Part model, mm, in its own coordinate system. A direction names the side the tool comes from. Coordinates: 2 decimals unless noted, no trailing zeros. Loops run counter-clockwise (first coordinate to the right, second up) from the corner with the lowest first, then second, coordinate; pieces in that order, holes last. Notation, with made-up numbers: M 72,22.5 L 119,22.5 A29 cw 119,46.5 Z; hole C 20.5,55 d11. An arc over 180 degrees is marked long. Use a Markdown table: item, result. Add a question column.
1) Band-saw the part on B-B (z = 0). State how many separate pieces and enclosed holes the cut face has, plus the area to 3 significant figures.
2) Band-saw the part on C-C (x = 6). List the corners of the cut face in (y, z) (3 decimals).
3) Tool access for faces 5 (the flat face through (-6.2, 8.094, 1.2)), 6 (the flat face through (-10, -3, 2)), 7 (the flat face through (1.3, 16, 13)), 8 (the cylindrical face through (0.659, 13.143, -17.141)), 9 (the flat face through (0, 9, 0)): list every direction of +Z, -Z, +X, -X, +Y, -Y with a clear straight run to the whole face (end or side of a thin tool).
4) Band-saw the part on A-A (x = -5). List the corners of the cut face in (y, z) (3 decimals).
5) Wall check: probe 1 along Y at (x, z) = (-3, 0) (3 decimals); probe 2 along X at (y, z) = (6.9, 0); probe 3 along Y at (x, z) = (1.5, 0) (3 decimals). Give the ranges that are in metal, low to high. Write a range as from..to.
6) Pull direction Z, two halves, no side cores. Call faces 1 (the cylindrical face through (21.659, 13.143, -17.141)), 2 (the conical face through (23.146, 3.144, -0.698)), 3 (the flat face through (22.3, 16, 13)), 4 (the cylindrical face through (-4.55, 5.43, 1.43)): released by +Z, released by -Z, zero draft, split by the parting line, or undercut.
7) Pin check, flat tips, straight feed: pin 1 Ø3.5 at (x, z) = (-5, 0) entering from +Y; pin 2 Ø3 at (x, y) = (8, 10.5) entering from -Z; pin 3 Ø5 at (y, z) = (-15.5, -16) entering from -X; pin 4 Ø5 at (y, z) = (0, 0) entering from +X. Stop position of each tip, or through.
from build123d import *

# Parameters (mm, degrees)
FILLET3_R               = 8
FILLET4_R               = 8
SKETCH3_W               = 12
SKETCH3_H               = 3.642473792
CUT_EXTRUDE1_DEPTH      = 10
CUT_EXTRUDE2_REACH      = 46.992
CUT_EXTRUDE2_END_RADIUS = 3.075
SKETCH4_R               = 1.5
CHAMFER1_SIZE           = 3


with BuildPart() as part:
    # Sketch1 → Revolve1 (revolve)
    with BuildSketch(Plane.XY, mode=Mode.PRIVATE) as revolve1_sk:
        Polygon((0, 21.6), (1.3, 21.6), (1.3, 20.2), (3.7, 20.2), (3.7, 21.6), (5, 21.6), (5, 13.075), (21, 13.075), (21, 21.6), (22.3, 21.6), (22.3, 20.2), (24.7, 20.2), (24.7, 21.6), (26, 21.6), (26, 3.075), (-10, 3.075), (-10, 10.075), (0, 10.075), align=None)
    revolve(revolve1_sk.sketch.rotate(Axis((0, 0, 0), (1, 0, 0)), 90), axis=Axis((0, 0, 0), (1, 0, 0)))

    # Fillet3
    fillet3_edges = [part.edges().sort_by_distance(p)[0] for p in [
        (5, 0, -13.075),
    ]]
    fillet(fillet3_edges, radius=FILLET3_R)

    # Fillet4
    fillet4_edges = [part.edges().sort_by_distance(p)[0] for p in [
        (21, 0, -13.075),
    ]]
    fillet(fillet4_edges, radius=FILLET4_R - 0.0001)  # a hair under: the kernel refuses the full size

    # Sketch3 → Cut-Extrude1 (cut)
    with BuildSketch(Plane.ZY.offset(10)):
        with Locations((0, 9.91479143)):
            Rectangle(SKETCH3_W, SKETCH3_H)
    extrude(amount=-CUT_EXTRUDE1_DEPTH, mode=Mode.SUBTRACT)

    # Cut-Extrude2: up to this cylinder (the profile starts outside it)
    cut_extrude2_end = Plane(origin=(-5, 0, 0), z_dir=(-1, 0, 0)) * Cylinder(CUT_EXTRUDE2_END_RADIUS, 101.134, mode=Mode.PRIVATE)
    # Sketch4 → Cut-Extrude2 (cut, up to the surface)
    with BuildSketch(Plane(origin=(0, 8.093554534, 0), x_dir=(1, 0, 0), z_dir=(0, 1, 0)), mode=Mode.PRIVATE) as cut_extrude2_sk1:
        with Locations(Location((-5, 0, 0), (0, 0, 270))):
            Circle(SKETCH4_R)
    cut_extrude2_tool1 = extrude(cut_extrude2_sk1.sketch, amount=-CUT_EXTRUDE2_REACH, mode=Mode.PRIVATE) - cut_extrude2_end
    add(cut_extrude2_tool1.solids().sort_by_distance((-5, 8.093555, 0))[0], mode=Mode.SUBTRACT)

    # Chamfer1
    chamfer1_edges = [part.edges().sort_by_distance(p)[0] for p in [
        (26, 0, -3.075),
    ]]
    chamfer(chamfer1_edges, length=CHAMFER1_SIZE)


solid = part.part
Entries:
| question | item | result |
|---|---|---|
| 1 | separate pieces | 3 |
| 1 | enclosed holes | 0 |
| 1 | area | 828 mm2 |
| 2 | outline | C 0,0 d34.404; hole C 0,0 d6.15 |
| 3 | face 5 | +Z, -Z, -X, +Y |
| 3 | face 6 | +Z, -Z, -X, +Y, -Y |
| 3 | face 7 | none |
| 3 | face 8 | +X, -X |
| 3 | face 9 | -X |
| 4 | outline | M 2.684,-1.5 A3.075 cw long 2.684,1.5 L 8.094,1.5 L 8.094,6 A10.075 ccw long 8.094,-6 L 8.094,-1.5 Z |
| 5 | probe 1 | -10.075..-3.075, 3.075..8.094 |
| 5 | probe 2 | -10..-6.5, -3.5..26 |
| 5 | probe 3 | -20.2..-3.075, 3.075..20.2 |
| 6 | face 1 | split by the parting line |
| 6 | face 2 | undercut |
| 6 | face 3 | zero draft |
| 6 | face 4 | undercut |
| 7 | pin 1 | y = 8.09 |
| 7 | pin 2 | z = -12.88 |
| 7 | pin 3 | x = 0 |
| 7 | pin 4 | through |
